Autodesk Inventor part; units mm, degrees
ref_plane "YZ Plane" through (0, 0, 0) normal (1, 0, 0) x (0, 1, 0)
ref_plane "XZ Plane" through (0, 0, 0) normal (0, 1, 0) x (-1, 0, 0)
ref_plane "XY Plane" through (0, 0, 0) normal (0, 0, 1) x (1, 0, 0)
sketch "Sketch1" plane through (0, 0, 0) normal (0, 0, 1) x (1, 0, 0)
  line L0 (-10, 10) -> (10, 10)
  line L1 (10, 10) -> (10, -10)
  line L2 (10, -10) -> (-10, -10)
  line L3 (-10, -10) -> (-10, 10)
  point P0 (0, 0)
  dimension "d0" = 20
  dimension "d1" = 20
  dimension "d2" = 10
  dimension "d3" = 10
extrude "Extrusion1" add sketch "Sketch1" along normal blind 300
sketch "Sketch2" plane through (-10, -10, 0) normal (-1, 0, 0) x (0, 0, 1)
  line L0 (0, 0) -> (0, 20)
  arc A0 (0, 20) -> (0, 0) centre (0, 10) ccw
extrude "Extrusion2" add sketch "Sketch2" against normal up to surface (20 mm away)
sketch "Sketch3" plane through (-10, -10, 300) normal (-1, 0, 0) x (0, 0, 1)
  circle A0 centre (-300, 10) radius 5
  dimension "d8" = 10
extrude "Extrusion3" cut sketch "Sketch3" against normal blind 30
properties part number "prismaticLink" material "Stainless Steel"
Can you work these out from the model? Positions are in its coordinate system, mm. Round coordinates to 2 decimals unless told otherwise and drop trailing zeros. Write each loop counter-clockwise with the first axis right and the second up, starting at its lowest first coordinate (ties: lowest second). Pieces come first, ordered by that corner, then holes. Notation, with made-up numbers: (14, -39) - (53, -39) arc R22 ccw to (53, -21) - close; hole circle Ø8 at (53.25, -1). An arc over 180 degrees is marked (long way). Write each question's results on one line, items separated by ' | '. Start each with the question number.
1) Suppose I cut it at A-A (y = 0). List the corners of the cut face in (x, z) for me, and give its area (3 significant figures).
2) Suppose I cut it at B-B (x = -3.5). List the corners of the cut face in (y, z) for me, and give its area (3 significant figures).
3) Please list where these lines run through material, in increasing order: line 1 (Y direction, x = 2, z = 0); line 2 (Z direction, x = -4.75, y = -3.5); line 3 (Z direction, x = -8, y = -3).
4) For pin 1 Ø6 at (x, y) = (3, 7.5) entering from -Z, with a flat end and sliding along its axis, tell me the tip position at first contact or that it passes through.
5) We'd pull the mould along Y, two halves only. Please class faces 1 (the flat face through (0, 0, 300)), 2 (the cylindrical face through (-0.14, -4.88, -1.08)), 3 (the flat face through (0, -10, 148)), 4 (the cylindrical face through (0, 0, -10)): released by +Y, released by -Y, zero draft, split by the parting line, or undercut.
Here are the results:
1) outline: (-10, -10) - (10, -10) - (10, -5) - (-10, -5) - close; (-10, 5) - (10, 5) - (10, 300) - (-10, 300) - close | area: 6,000 mm2
2) outline: (-10, 0) arc R10 ccw to (10, 0) - (10, 300) - (-10, 300) - close; hole circle Ø10 at (0, 0) | area: 6,080 mm2
3) line 1: y = -10 to -5, 5 to 10 | line 2: z = -9.37 to -3.57, 3.57 to 300 | line 3: z = -9.54 to -4, 4 to 300
4) pin 1: stops at z = -8.93
5) face 1: zero draft | face 2: undercut | face 3: released by -Y | face 4: split by the parting line
